from build123d import *

# Parameters (mm, degrees)
BOSS_EXTRUDE1_DEPTH = 90
SKETCH3_W           = 90
SKETCH3_H           = 11.4
BOSS_EXTRUDE3_DEPTH = 47.5
SKETCH6_R           = 5.5
CUT_EXTRUDE3_DEPTH  = 5.5
SKETCH7_R           = 2.8
CUT_EXTRUDE4_DEPTH  = 10
BOSS_EXTRUDE4_DEPTH = 90


with BuildPart() as part:
    # Sketch1 → Boss-Extrude1 (new body)
    with BuildSketch(Plane(origin=(0, 0, 0), x_dir=(0, 0, -1), z_dir=(1, 0, 0))):
        Polygon((-16.5, 7.5), (16.5, 7.5), (16.5, -15), (6.5, -15), (6.5, -10), (10.5, -10), (10.5, -2.5), (3, -2.5), (3, -7.7), (-3, -7.7), (-3, -2.5), (-10.5, -2.5), (-10.5, -10), (-6.5, -10), (-6.5, -15), (-16.5, -15), align=None)
    extrude(amount=BOSS_EXTRUDE1_DEPTH)

    # Sketch3 → Boss-Extrude3 (add)
    with BuildSketch(Plane(origin=(0, 7.5, 0), x_dir=(1, 0, 0), z_dir=(0, 1, 0))):
        with Locations((45, 10.8)):
            Rectangle(SKETCH3_W, SKETCH3_H)
    extrude(amount=BOSS_EXTRUDE3_DEPTH)

    # Sketch6 → Cut-Extrude3 (cut)
    with BuildSketch(Plane(origin=(0, 0, -16.5), x_dir=(-1, 0, 0), z_dir=(0, 0, -1))):
        with Locations((-70, 45)):
            Circle(SKETCH6_R)
        with Locations((-20, 45)):
            Circle(SKETCH6_R)
    extrude(amount=-CUT_EXTRUDE3_DEPTH, mode=Mode.SUBTRACT)

    # Sketch7 → Cut-Extrude4 (cut)
    with BuildSketch(Plane(origin=(0, 0, -11), x_dir=(-1, 0, 0), z_dir=(0, 0, -1))):
        with Locations((-70, 45)):
            Circle(SKETCH7_R)
        with Locations((-20, 45)):
            Circle(SKETCH7_R)
    extrude(amount=-CUT_EXTRUDE4_DEPTH, mode=Mode.SUBTRACT)

    # Sketch11 → Boss-Extrude4 (add)
    with BuildSketch(Plane.ZY):
        Polygon((-5.1, 17.5), (4.9, 7.5), (-5.1, 7.5), align=None)
    extrude(amount=-BOSS_EXTRUDE4_DEPTH)


solid = part.part
Source: CAD feature listing. Evaluate the final solid. Frame: model axes, mm. A direction names the side the tool comes from. Coordinates: 2 decimals unless noted, no trailing zeros. Loops run counter-clockwise (first coordinate to the right, second up) from the corner with the lowest first, then second, coordinate; pieces in that order, holes last. Notation, with made-up numbers: (77, 41) - (114, 41) arc R16 cw to (114, 50) - close; hole circle Ø3 at (-17, -17.75). An arc over 180 degrees is marked (long way). One line per item, written item: value. Start each with the question number.
1. Section B-B (z = 8). Return the cut outline in (x, y).
2. Ray query, L1, parallel to Y at x = 20, z = -8; L2, parallel to Y at x = 20, z = -14.3; L3, parallel to Y at x = 42.5, z = -10. Return the intervals inside material, ascending.
3. Contact query for flat-ended pins moving along their axis: P1, Ø3, axis at x = 49.5, z = 9, coming from the +Y side; P2, Ø5, axis at x = 49, z = -1, coming from the -Y side; P3, Ø6, axis at x = 28.5, y = 38.5, coming from the +Z side; P4, Ø4, axis at y = 10.5, z = 10.5, coming from the +X side. Output: stop coordinate, or through.
4. Section D-D (x = 57.5). Return the cut outline in (y, z), and give its area (3 significant figures).
5. Mould query, pull axis Y, two halves, no side actions, for faces 1 (the flat face through (44, 7.5, 11)), 2 (the flat face through (23, 46, -11)), 3 (the flat face through (44, -7.7, 0)). Classes: pulls with the +Y half, pulls with the -Y half, needs draft (parallel to the pull), parting line crosses it, or undercut.
6. Section A-A (x = 20). Return the cut outline in (y, z), and give its area (3 significant figures).
7. Section C-C (y = 45). Return the cut outline in (x, z).
8. Set-up query: faces 4 (the cylindrical face through (75.495, 45.242, -13.788)), 5 (the flat face through (44, -13, -6.5)), 6 (the flat face through (44, -10, -8)). Return all of +Z, -Z, +X, -X, +Y, -Y with unobstructed straight access to the full face (end or side cutting, diameter ignored); none if empty.
Verdict:
1. outline: (0, -15) - (90, -15) - (90, -10) - (0, -10) - close; (0, -2.5) - (90, -2.5) - (90, 7.5) - (0, 7.5) - close
2. L1: y = -15 to -10, -2.5 to 42.2, 47.8 to 55
2. L2: y = -15 to 39.5, 50.5 to 55
2. L3: y = -15 to -10, -2.5 to 55
3. P1: stops at y = 7.5
3. P2: stops at y = -7.7
3. P3: stops at z = -5.1
3. P4: passes through
4. outline: (-15, -16.5) - (55, -16.5) - (55, -5.1) - (17.5, -5.1) - (7.5, 4.9) - (7.5, 16.5) - (-15, 16.5) - (-15, 6.5) - (-10, 6.5) - (-10, 10.5) - (-2.5, 10.5) - (-2.5, 3) - (-7.7, 3) - (-7.7, -3) - (-2.5, -3) - (-2.5, -10.5) - (-10, -10.5) - (-10, -6.5) - (-15, -6.5) - close
4. area: 1,140 mm2
5. face 1: pulls with the +Y half
5. face 2: undercut
5. face 3: pulls with the -Y half
6. outline: (-15, -16.5) - (39.5, -16.5) - (39.5, -11) - (42.2, -11) - (42.2, -5.1) - (17.5, -5.1) - (7.5, 4.9) - (7.5, 16.5) - (-15, 16.5) - (-15, 6.5) - (-10, 6.5) - (-10, 10.5) - (-2.5, 10.5) - (-2.5, 3) - (-7.7, 3) - (-7.7, -3) - (-2.5, -3) - (-2.5, -10.5) - (-10, -10.5) - (-10, -6.5) - (-15, -6.5) - close; (47.8, -11) - (50.5, -11) - (50.5, -16.5) - (55, -16.5) - (55, -5.1) - (47.8, -5.1) - close
6. area: 1,050 mm2
7. outline: (0, -16.5) - (14.5, -16.5) - (14.5, -11) - (17.2, -11) - (17.2, -5.1) - (0, -5.1) - close; (22.8, -11) - (25.5, -11) - (25.5, -16.5) - (64.5, -16.5) - (64.5, -11) - (67.2, -11) - (67.2, -5.1) - (22.8, -5.1) - close; (72.8, -11) - (75.5, -11) - (75.5, -16.5) - (90, -16.5) - (90, -5.1) - (72.8, -5.1) - close
8. face 4: -Z
8. face 5: +X, -X, -Y
8. face 6: +X, -X
